The figure shows three views and two pictorial views of one solid part (mm, origin at its lowest corner). Answer the questions. A direction names the side the tool comes from. Coordinates: 2 decimals unless noted, no trailing zeros. Order: outer loops, then holes, each group sorted by start corner. A loop starts at its lowest first (then second) coordinate and runs counter-clockwise, first axis right, second up. Notation, with made-up numbers: (10, -31.75) - (30, -31.75) arc R30 ccw to (30, 3.25) - close; hole circle Ø3 at (77.5, -28). An arc over 180 degrees is marked (long way). Answer as a JSON object with one key per item and string values. Group by question number.
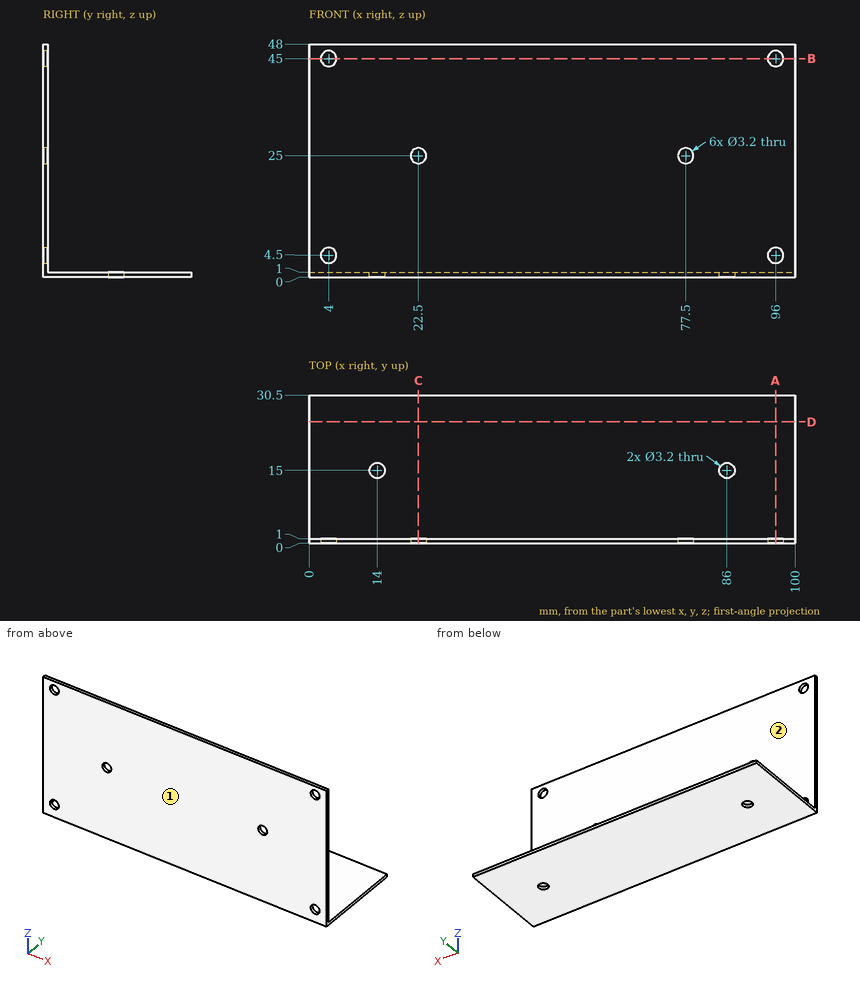
1. A cutting plane is placed at B-B on z = 45. Write down the section's boundary in (x, y), and give its area (3 significant figures).
2. Given pin 1 (12 mm diameter, centred on y = 21.5, z = 12.5, fed in from -X); pin 2 (3 mm diameter, centred on x = 29.5, y = 3.5, fed in from +Z); pin 3 (3 mm diameter, centred on x = 61.5, z = 23.5, fed in from +Y), each flat-ended and moving along its own axis, determine where each tip first touches the part or whether it passes through.
3. A cutting plane is placed at D-D on y = 25. Write down the section's boundary in (x, z), and give its area (3 significant figures).
4. A cutting plane is placed at C-C on x = 22.5. Write down the section's boundary in (y, z).
5. For the marked faces 1 and 2, determine the directions among +Z, -Z, +X, -X, +Y, -Y from which every point of the face is accessible in a straight line to the end or side of a thin tool.
6. A cutting plane is placed at A-A on x = 96. Write down the section's boundary in (y, z).
7. Straight lines are drawn through the part: L1, parallel to X at y = 0.3, z = 45; L2, parallel to Z at x = 24.5, y = 7. For each, find the intervals that lie inside material, in ascending order.
Derived:
{
 "1": {"outline": "(0, 0) - (2.4, 0) - (2.4, 1) - (0, 1) - close; (5.6, 0) - (94.4, 0) - (94.4, 1) - (5.6, 1) - close; (97.6, 0) - (100, 0) - (100, 1) - (97.6, 1) - close", "area": "93.6 mm2"},
 "2": {"pin 1": "passes through", "pin 2": "stops at z = 1", "pin 3": "stops at y = 1"},
 "3": {"outline": "(0, 0) - (100, 0) - (100, 1) - (0, 1) - close", "area": "100 mm2"},
 "4": {"outline": "(0, 0) - (30.5, 0) - (30.5, 1) - (1, 1) - (1, 23.4) - (0, 23.4) - close; (0, 26.6) - (1, 26.6) - (1, 48) - (0, 48) - close"},
 "5": {"face 1": "+Z, -Z, +X, -X, -Y", "face 2": "+Z, +X, -X, +Y"},
 "6": {"outline": "(0, 0) - (30.5, 0) - (30.5, 1) - (1, 1) - (1, 2.9) - (0, 2.9) - close; (0, 6.1) - (1, 6.1) - (1, 43.4) - (0, 43.4) - close; (0, 46.6) - (1, 46.6) - (1, 48) - (0, 48) - close"},
 "7": {"L1": "x = 0 to 2.4, 5.6 to 94.4, 97.6 to 100", "L2": "z = 0 to 1"}
}
